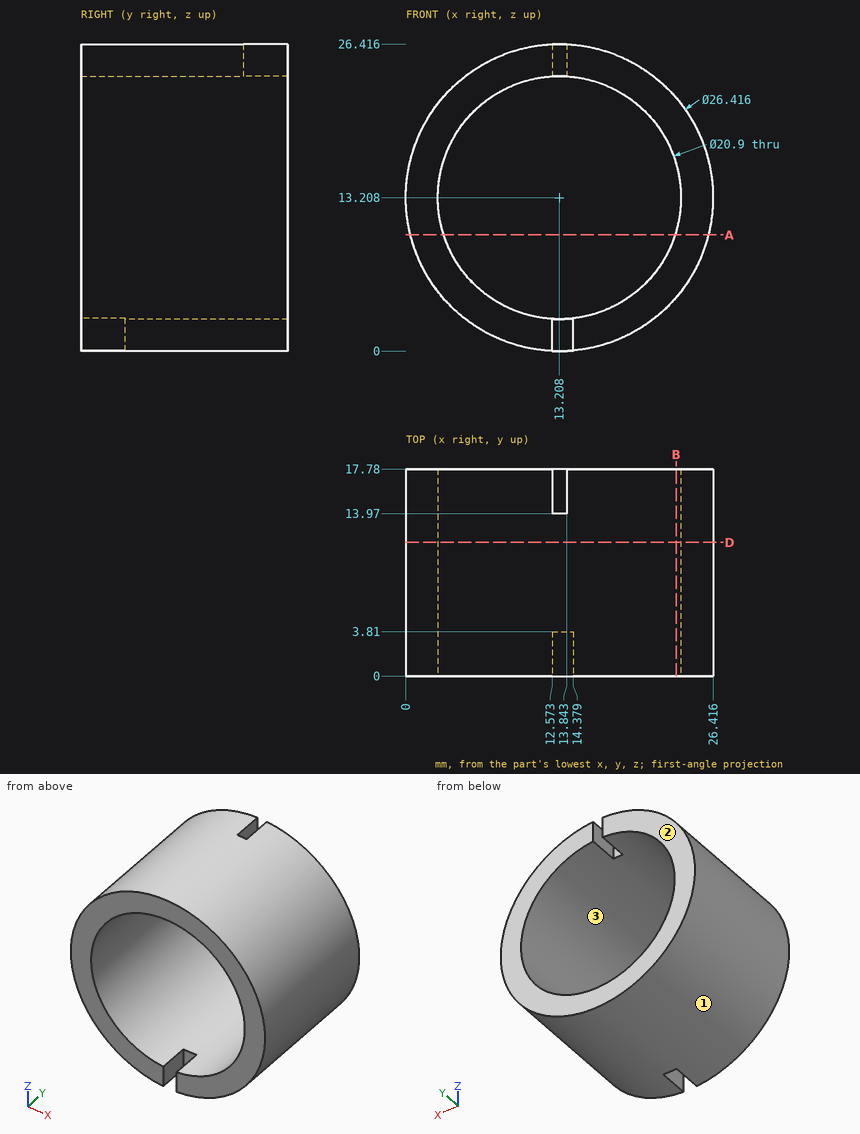
Can you work these out from the drawing? Everything is in mm from the part's minimum corner. Coordinates: 2 decimals unless noted, no trailing zeros. Write each loop counter-clockwise with the first axis right and the second up, starting at its lowest first coordinate (ties: lowest second). Pieces come first, ordered by that corner, then holes. Notation, with made-up numbers: (81.5, -32.5) -> (133.5, -32.5) arc R16 ccw to (133.5, -21.5) -> close; hole circle Ø2 at (-5.5, 49.25). An arc over 180 degrees is marked (long way). Return JSON: item names as keys, results as strings.
(1) I need wall thicknesses on L1, parallel to X at y = 16, z = 12.5 (1 decimal); L2, parallel to Z at x = 5, y = 16 (1 decimal); L3, parallel to Z at x = 21, y = 13.5 (1 decimal). Which ranges of each line are inside material? Lowest first, please.
Numbers:
{"L1": "x = 0 to 2.8, 23.6 to 26.4", "L2": "z = 2.9 to 6.7, 19.7 to 23.6", "L3": "z = 2.5 to 6.2, 20.2 to 23.9"}
(2) I'm going to push flat-ended pins straight in: pin 1 (3 mm diameter, centred on y = 15.5, z = 25.5, fed in from -X) (1 decimal); pin 2 (2 mm diameter, centred on y = 1, z = 1.5, fed in from -X) (1 decimal); pin 3 (5 mm diameter, centred on x = 4.5, y = 3, fed in from -Z). Where does each tip first touch, or does it pass through?
Numbers:
{"pin 1": "stops at x = 5.6", "pin 2": "stops at x = 5.5", "pin 3": "stops at z = 1.55"}
(3) Imagine slicing it at D-D, the plane y = 11.5. Please give me the cut outline in (x, z).
Numbers:
{"outline": "circle Ø26.42 at (13.21, 13.21); hole circle Ø20.9 at (13.21, 13.21)"}
(4) Imagine slicing it at B-B, the plane x = 23.25. Please give me the cut outline in (y, z).
Numbers:
{"outline": "(0, 4.63) -> (17.78, 4.63) -> (17.78, 10.32) -> (0, 10.32) -> close; (0, 16.1) -> (17.78, 16.1) -> (17.78, 21.79) -> (0, 21.79) -> close"}
(5) Imagine slicing it at A-A, the plane z = 10. Please give me the cut outline in (x, y) (1 decimal), then the cut area to 3 significant figures.
Numbers:
{"outline": "(0.4, 0) -> (3.3, 0) -> (3.3, 17.8) -> (0.4, 17.8) -> close; (23.2, 0) -> (26, 0) -> (26, 17.8) -> (23.2, 17.8) -> close", "area": "102 mm2"}
(6) We'd pull the mould along Z, two halves only. Please class the marked faces 1, 2 and 3: +Z half, -Z half, draft (parallel to the pull), parting line (faces both ways), or undercut.
Numbers:
{"face 1": "parting line", "face 2": "draft", "face 3": "undercut"}
